from build123d import *

# Parameters (mm, degrees)
SKETCH1_W           = 300
SKETCH1_H           = 400
SKETCH1_R           = 4
BOSS_EXTRUDE1_DEPTH = 25


with BuildPart() as part:
    # Sketch1 → Boss-Extrude1 (new body)
    with BuildSketch(Plane.XY):
        Rectangle(SKETCH1_W, SKETCH1_H)
        with Locations((-112, -170)):
            Circle(SKETCH1_R, mode=Mode.SUBTRACT)
        with Locations((-140, -170)):
            Circle(SKETCH1_R, mode=Mode.SUBTRACT)
        with Locations(Location((112, -170, 0), (0, 0, 180))):
            Circle(SKETCH1_R, mode=Mode.SUBTRACT)
        with Locations(Location((140, -170, 0), (0, 0, 180))):
            Circle(SKETCH1_R, mode=Mode.SUBTRACT)
        with Locations((112, -30)):
            Circle(SKETCH1_R, mode=Mode.SUBTRACT)
        with Locations((140, -30)):
            Circle(SKETCH1_R, mode=Mode.SUBTRACT)
        with Locations(Location((-112, -30, 0), (0, 0, 180))):
            Circle(SKETCH1_R, mode=Mode.SUBTRACT)
        with Locations(Location((-140, -30, 0), (0, 0, 180))):
            Circle(SKETCH1_R, mode=Mode.SUBTRACT)
    extrude(amount=-BOSS_EXTRUDE1_DEPTH)


solid = part.part
Part model, mm, in its own coordinate system. Give positions to 0.01 mm unless a question says otherwise; leave off trailing zeros. Write each question's results on one line, items separated by ' | '. Start each with the question number.
Q1. Pin check, flat tip, straight feed: P1, Ø10.5, axis at x = 140, y = -170, coming from the +Z side. Stop position of the tip, or through.
Q2. Wall check: L1, parallel to Y at x = -112, z = -18.25. Give the ranges that are in metal, low to high.
Q3. Pull direction X, two halves, no side cores. Call faces 1 (the face through (-143.815, -31.201, -12.325)), 2 (the face through (-2, 3, 0)), 3 (the face through (150, -3, -12)): +X half, -X half, draft (parallel to the pull), parting line (faces both ways), or undercut.
Results are:
1) P1: stops at z = 0
2) L1: y = -200 to -174, -166 to -34, -26 to 200
3) face 1: undercut | face 2: draft | face 3: +X half
